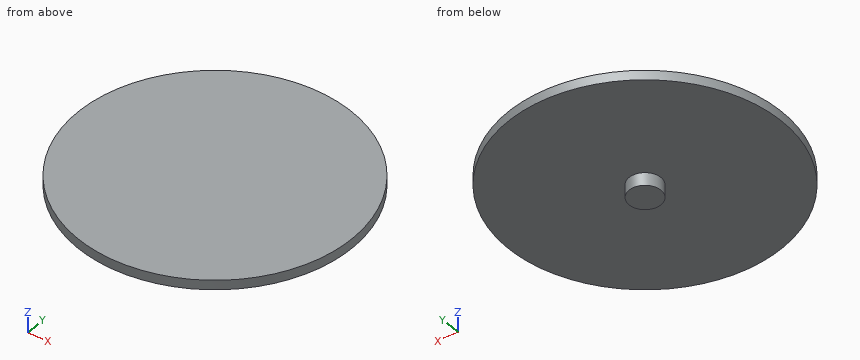
```python
from build123d import *

# Parameters (mm, degrees)
EXTRUDE_START      = 317
EXTRUDE_SKETCH_1_R = 86
EXTRUDE_1_DEPTH    = 6
EXTRUDE_START_2    = 309
EXTRUDE_SKETCH_2_R = 10
EXTRUDE_2_DEPTH    = 8


with BuildPart() as part:
    # Extrude sketch 1 → Extrude 1 (new body)
    with BuildSketch(Plane.XY.offset(EXTRUDE_START)):
        with Locations((757.5, 0)):
            Circle(EXTRUDE_SKETCH_1_R)
    extrude(amount=EXTRUDE_1_DEPTH)


with BuildPart() as body_2:
    # Extrude sketch 2 → Extrude 2 (new body)
    with BuildSketch(Plane.XY.offset(EXTRUDE_START_2)):
        with Locations((757.5, 0)):
            Circle(EXTRUDE_SKETCH_2_R)
    extrude(amount=EXTRUDE_2_DEPTH)


with BuildPart() as part_1:
    add(part.part)

    # Combine (weld / assembly of features): union body 2
    add(body_2.part)


solid = part_1.part
```
The listing builds one solid part. Answer for the finished solid, in the listing's coordinates (mm). Coordinates: 2 decimals unless noted, no trailing zeros. Loops run counter-clockwise (first coordinate to the right, second up) from the corner with the lowest first, then second, coordinate; pieces in that order, holes last. Notation, with made-up numbers: (3, 38) -> (23, 38) arc R26 cw to (23, 72) -> close; hole circle Ø9 at (28.25, 23.5). An arc over 180 degrees is marked (long way). Use one line per item in the form item = value. Start each with the question number.
Item 1: The part is cut by section A-A on y = 0. Determine the outline of the cut face in (x, z).
Item 2: The part is cut by section B-B on x = 757.5. Determine the outline of the cut face in (y, z), then the cut area to 3 significant figures.
Item 3: Consider L1, parallel to Z at x = 819, y = -43.5; L2, parallel to Y at x = 699.5, z = 318.25; L3, parallel to X at y = -59, z = 320.5. Determine where each line is inside the solid, lowest interval first. Write a range as [from, to].
Item 4: The part is cut by section C-C on z = 313. Determine the outline of the cut face in (x, y), then the cut area to 3 significant figures.
Item 5: Flat-ended cylindrical pins translate along their axes: pin 1 Ø10 at (x, y) = (746, -37.5) entering from -Z; pin 2 Ø3 at (x, z) = (817, 314) entering from -Y. Find the tip coordinate at first contact, or state that the pin passes through.
Item 6: The part is cut by section D-D on x = 806. Determine the outline of the cut face in (y, z).
Answer key:
q1.outline = (671.5, 317) -> (747.5, 317) -> (747.5, 309) -> (767.5, 309) -> (767.5, 317) -> (843.5, 317) -> (843.5, 323) -> (671.5, 323) -> close
q2.outline = (-86, 317) -> (-10, 317) -> (-10, 309) -> (10, 309) -> (10, 317) -> (86, 317) -> (86, 323) -> (-86, 323) -> close
q2.area = 1,190 mm2
q3.L1 = [317, 323]
q3.L2 = [-63.5, 63.5]
q3.L3 = [694.93, 820.07]
q4.outline = circle Ø20 at (757.5, 0)
q4.area = 314 mm2
q5.pin_1 = 317
q5.pin_2 = through
q6.outline = (-71.02, 317) -> (71.02, 317) -> (71.02, 323) -> (-71.02, 323) -> close
